```python
from build123d import *

# Parameters (mm, degrees)
F0_R     = 90
F1_DEPTH = 2.5


with BuildPart() as f1:
    # F0 (on Front) → F1 (new body, symmetric)
    with BuildSketch(Plane.XZ):
        with BuildLine():
            Line((130, 275), (-130, 275))
            ThreePointArc((-130, 275), (-144.142136, 269.142136), (-150, 255))
            Line((-150, 255), (-150, -255))
            ThreePointArc((-150, -255), (-144.142136, -269.142136), (-130, -275))
            Line((-130, -275), (130, -275))
            ThreePointArc((130, -275), (144.142136, -269.142136), (150, -255))
            Line((150, -255), (150, 255))
            ThreePointArc((150, 255), (144.142136, 269.142136), (130, 275))
        make_face()
        with Locations((0, -75)):
            Circle(F0_R, mode=Mode.SUBTRACT)
    extrude(amount=F1_DEPTH, both=True)


solid = f1.part
```
Build history of the part. All positions in model axes, mm. Round coordinates to 2 decimals unless told otherwise and drop trailing zeros. Loops run counter-clockwise (first coordinate to the right, second up) from the corner with the lowest first, then second, coordinate; pieces in that order, holes last.
Item 1: Two-plate mould, pull along X, no slides. Class faces 1 (the face through (-2, 2.5, 65)), 2 (the face through (85.844, 0.035, -47.966)), 3 (the face through (144.297, -0.035, 268.986)), 4 (the face through (-144.297, -0.035, -268.986)): released by +X, released by -X, zero draft, split by the parting line, or undercut.
Item 2: Saw through at A-A (x = 0). List the corners of the cut face in (y, z).
Item 3: Saw through at B-B (y = -0.2). List the corners of the cut face in (x, z), then the cut area to 3 significant figures.
Item 4: Drill centre lines: line 1 along X through (y, z) = (1.85, -79); line 2 along Z through (x, y) = (0, -0.25); line 3 along Z through (x, y) = (-56.5, 2.25). Where is each one in solid material? Low to high.
Item 5: Saw through at C-C (z = -75). List the corners of the cut face in (x, y).
Worked answers:
1. face 1: zero draft
1. face 2: undercut
1. face 3: released by +X
1. face 4: released by -X
2. outline: (-2.5, -275) - (2.5, -275) - (2.5, -165) - (-2.5, -165) - close; (-2.5, 15) - (2.5, 15) - (2.5, 275) - (-2.5, 275) - close
3. outline: (-150, -255) arc R20 ccw to (-130, -275) - (130, -275) arc R20 ccw to (150, -255) - (150, 255) arc R20 ccw to (130, 275) - (-130, 275) arc R20 ccw to (-150, 255) - close; hole circle Ø180 at (0, -75)
3. area: 139,000 mm2
4. line 1: x = -150 to -89.91, 89.91 to 150
4. line 2: z = -275 to -165, 15 to 275
4. line 3: z = -275 to -145.06, -4.94 to 275
5. outline: (-150, -2.5) - (-90, -2.5) - (-90, 2.5) - (-150, 2.5) - close; (90, -2.5) - (150, -2.5) - (150, 2.5) - (90, 2.5) - close
